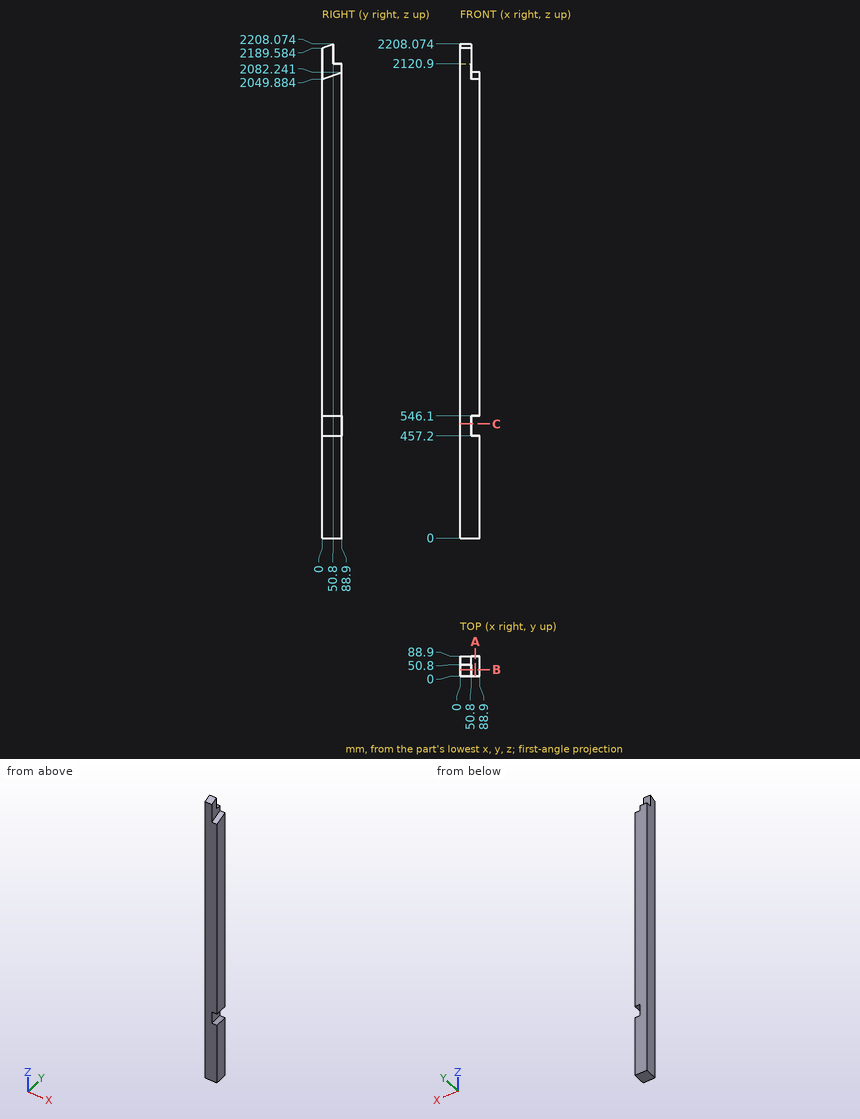
Study the drawing (mm; zero at the part's minimum x, y, z) and answer. Coordinates: 2 decimals unless noted, no trailing zeros. Order: outer loops, then holes, each group sorted by start corner. A loop starts at its lowest first (then second) coordinate and runs counter-clockwise, first axis right, second up. Notation, with made-up numbers: M -4,67.5 L 42,67.5 A21 cw 42,96.5 Z; hole C 31,-10.75 d2. An arc over 180 degrees is marked long. Answer as a JSON object with one key per item and string values. Group by question number.
1. Section B-B on y = 29 is taken. Write down the section's boundary in (x, z), then the cut area to 3 significant figures.
2. A flat-ended cylindrical pin translates along its axis: P1, Ø19, axis at x = 69.5, y = 48, coming from the +Z side. Find the tip coordinate at first contact, or state that the pin passes through.
3. Section A-A on x = 68.5 is taken. Write down the section's boundary in (y, z), then the cut area to 3 significant figures.
4. Straight lines are drawn through the part: line 1 (Z direction, x = 45, y = 62); line 2 (Z direction, x = 83, y = 20.5) (1 decimal); line 3 (Z direction, x = 79, y = 66). For each, find the intervals that lie inside material, in ascending order.
5. Section C-C on z = 511 is taken. Write down the section's boundary in (x, y), then the cut area to 3 significant figures.
Values follow:
{
 "1": {"outline": "M 0,0 L 88.9,0 L 88.9,457.2 L 50.8,457.2 L 50.8,546.1 L 88.9,546.1 L 88.9,2060.44 L 50.8,2060.44 L 50.8,2200.14 L 0,2200.14 Z", "area": "187,000 mm2"},
 "2": {"P1": "z = 2070.81"},
 "3": {"outline": "M 0,0 L 88.9,0 L 88.9,457.2 L 0,457.2 Z; M 0,546.1 L 88.9,546.1 L 88.9,2082.24 L 0,2049.88 Z", "area": "176,000 mm2"},
 "4": {"line 1": "0 to 2120.9", "line 2": "0 to 457.2, 546.1 to 2057.3", "line 3": "0 to 457.2, 546.1 to 2073.91"},
 "5": {"outline": "M 0,0 L 50.8,0 L 50.8,88.9 L 0,88.9 Z", "area": "4,520 mm2"}
}
